Check sheet for the modelled part. Datum: model origin and axes. Units: mm. Face numbers are marked on the shaded views. Round coordinates to 2 decimals unless told otherwise and drop trailing zeros. Write each loop counter-clockwise with the first axis right and the second up, starting at its lowest first coordinate (ties: lowest second). Pieces come first, ordered by that corner, then holes. Notation, with made-up numbers: M 68,-13 L 87,-13 A17 ccw 87,-1 Z; hole C 75.25,29 d10. An arc over 180 degrees is marked long. One line per item, written item: value.
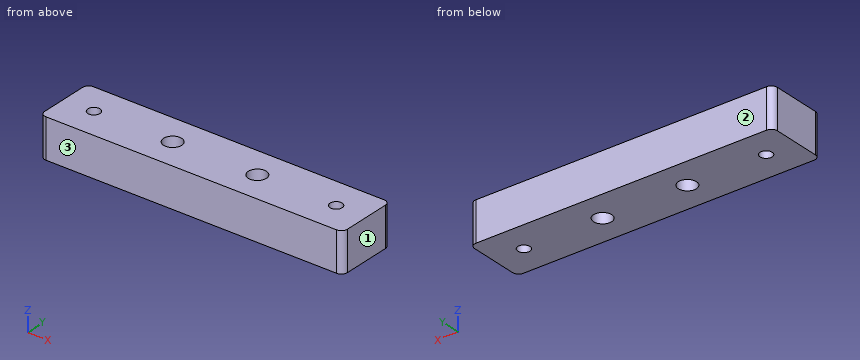
from build123d import *

# Parameters (mm, degrees)
SKETCH1_W           = 100
SKETCH1_H           = 20
BOSS_EXTRUDE1_DEPTH = 13
SKETCH2_R           = 3
SKETCH2_R_2         = 2
CUT_EXTRUDE1_DEPTH  = 13
CUT_EXTRUDE2_DEPTH  = 13


with BuildPart() as part:
    # Sketch1 → Boss-Extrude1 (new body)
    with BuildSketch(Plane.XY):
        with Locations((50, 10)):
            Rectangle(SKETCH1_W, SKETCH1_H)
    extrude(amount=BOSS_EXTRUDE1_DEPTH)

    # Sketch2 → Cut-Extrude1 (cut)
    with BuildSketch(Plane.XY.offset(13)):
        with Locations((64, 10)):
            Circle(SKETCH2_R)
        with Locations((36, 10)):
            Circle(SKETCH2_R)
        with Locations((10, 10)):
            Circle(SKETCH2_R_2)
        with Locations((90, 10)):
            Circle(SKETCH2_R_2)
    extrude(amount=-CUT_EXTRUDE1_DEPTH, mode=Mode.SUBTRACT)

    # Sketch3 → Cut-Extrude2 (cut)
    with BuildSketch(Plane.XY.offset(13)):
        with BuildLine():
            ThreePointArc((98, 20), (99.414213562, 19.414213562), (100, 18))
            Line((100, 18), (100, 20))
            Line((100, 20), (98, 20))
        make_face()
        with BuildLine():
            ThreePointArc((100, 2), (99.414213562, 0.585786438), (98, 0))
            Line((98, 0), (100, 0))
            Line((100, 0), (100, 2))
        make_face()
        with BuildLine():
            Line((0, 0), (2, 0))
            ThreePointArc((2, 0), (0.585786438, 0.585786438), (0, 2))
            Line((0, 2), (0, 0))
        make_face()
        with BuildLine():
            Line((0, 20), (0, 18))
            ThreePointArc((0, 18), (0.585786438, 19.414213562), (2, 20))
            Line((2, 20), (0, 20))
        make_face()
    extrude(amount=-CUT_EXTRUDE2_DEPTH, mode=Mode.SUBTRACT)


solid = part.part
Q1. Draft check along Y on the marked faces 1, 2 and 3. Enter one of: pulls with the +Y half, pulls with the -Y half, needs draft (parallel to the pull), parting line crosses it, or undercut.
Completed:
face 1: needs draft
face 2: pulls with the +Y half
face 3: pulls with the -Y half
Q2. Sectioned sample at C-C on z = 8.75. Enter the section's corners in (x, y), and give its area (3 significant figures).
Completed:
outline: M 0,2 A2 ccw 2,0 L 98,0 A2 ccw 100,2 L 100,18 A2 ccw 98,20 L 2,20 A2 ccw 0,18 Z; hole C 10,10 d4; hole C 36,10 d6; hole C 64,10 d6; hole C 90,10 d4
area: 1,910 mm^2
Q3. Sectioned sample at A-A on y = 10. Enter the section's corners in (x, z).
Completed:
outline: M 0,0 L 8,0 L 8,13 L 0,13 Z; M 12,0 L 33,0 L 33,13 L 12,13 Z; M 39,0 L 61,0 L 61,13 L 39,13 Z; M 67,0 L 88,0 L 88,13 L 67,13 Z; M 92,0 L 100,0 L 100,13 L 92,13 Z
Q4. Sectioned sample at D-D on x = 64. Enter the section's corners in (y, z).
Completed:
outline: M 0,0 L 7,0 L 7,13 L 0,13 Z; M 13,0 L 20,0 L 20,13 L 13,13 Z
Q5. Scan lines: line 1 (X direction, y = 9.75, z = 3.5); line 2 (Y direction, x = 90, z = 8.25); line 3 (X direction, y = 8.25, z = 6.5). Record each from-to range of solid material in increasing order. Write a range as [from, to].
Completed:
line 1: [0, 8.02], [11.98, 33.01], [38.99, 61.01], [66.99, 88.02], [91.98, 100]
line 2: [0, 8], [12, 20]
line 3: [0, 9.03], [10.97, 33.56], [38.44, 61.56], [66.44, 89.03], [90.97, 100]
Q6. Sectioned sample at B-B on x = 90. Enter the section's corners in (y, z), and give its area (3 significant figures).
Completed:
outline: M 0,0 L 8,0 L 8,13 L 0,13 Z; M 12,0 L 20,0 L 20,13 L 12,13 Z
area: 208 mm^2
